Read the model definition and answer for the solid it produces. Units are mm, in the model's axes. Face numbers are marked on the shaded views. A direction names the side the tool comes from. Give positions to 0.01 mm unless a question says otherwise; leave off trailing zeros. Write each loop counter-clockwise with the first axis right and the second up, starting at its lowest first coordinate (ties: lowest second). Pieces come first, ordered by that corner, then holes. Notation, with made-up numbers: (19.5, 74.5) - (29.5, 74.5) arc R20 ccw to (29.5, 83.5) - close; hole circle Ø3 at (23, 16.25). An arc over 180 degrees is marked (long way). Use CSV: the item, a comma, the result in double quotes. Start each with the question number.
from build123d import *

# Parameters (mm, degrees)
RIB1_REACH          = 71.607
SKETCH3_WALL_W      = 156.928914452
SKETCH3_WALL_H      = 8
CHAMFER1_SIZE       = 2
CHAMFER1_SIZE2      = 20
CHAMFER2_SIZE       = 1
CHAMFER2_SIZE2      = 1.144674394
CIRPATTERN23_COUNT  = 4
CUT_EXTRUDE7_REACH  = 71.607
SKETCH5_R           = 1
CIRPATTERN24_COUNT  = 4
SKETCH4_OUTSIDE_W   = 79.882
SKETCH4_OUTSIDE_H   = 79.882
SKETCH4_OUTSIDE_R   = 16.631613782
CUT_EXTRUDE8_DEPTH  = 20
CUT_EXTRUDE8_DRAFT  = -2
SKETCH7_OUTSIDE_W   = 78.484
SKETCH7_OUTSIDE_H   = 78.484
SKETCH7_OUTSIDE_W_2 = 54
SKETCH7_OUTSIDE_H_2 = 56.5
CUT_EXTRUDE9_DEPTH  = 57


with BuildPart() as part:
    # Sketch1 → Revolve1 (revolve)
    with BuildSketch(Plane(origin=(0, 0, 0), x_dir=(0, 0, -1), z_dir=(1, 0, 0))):
        Polygon((10.5, 57), (15.5, 57), (15.921613782, 36.013708049), (16.631613782, 36.013708049), (18.25, 6), (28.25, 6), (28.25, 0), (23.75, 0), (23.75, -3), (19.25, -3), (19.25, 0), (13.75, 0), (13.75, 6.707783598), (12.75, 6.707783598), (12.75, 8.013708049), (11.75, 8.013708049), (11.75, 36.013708049), (10.75, 36.013708049), (10.5, 53), align=None)
    revolve(axis=Axis((0, 0, 0), (0, 1, 0)))

    # Sketch3 wall → Rib1 (add, up to next)
    with BuildSketch(Plane(origin=(22.676470588, 12, 0), x_dir=(0.645690512921, -0.763599215245, 0), z_dir=(0.763599215245, 0.645690512921, 0)), mode=Mode.PRIVATE) as rib1_sk1:
        Rectangle(SKETCH3_WALL_W, SKETCH3_WALL_H)
    rib1_tool1 = extrude(rib1_sk1.sketch, amount=-RIB1_REACH, mode=Mode.PRIVATE) - part.part
    rib1 = rib1_tool1.solids().sort_by_distance((22.676470588, 12, 0))[0]
    add(rib1)

    # Chamfer1
    chamfer1_edges = [part.edges().sort_by_distance(p)[0] for p in [
        (0, 57, 15.5),
    ]]
    chamfer1_side = [part.faces().sort_by_distance(p)[0] for p in [
        (0, 57, 10.938406204),
    ]]
    chamfer(chamfer1_edges, length=CHAMFER1_SIZE, length2=CHAMFER1_SIZE2, reference=chamfer1_side[0])

    # Chamfer2
    chamfer2_edges = [part.edges().sort_by_distance(p)[0] for p in [
        (0, 57, 13.5),
    ]]
    chamfer2_side = [part.faces().sort_by_distance(p)[0] for p in [
        (0, 47.002017422, 14.700859078),
    ]]
    chamfer(chamfer2_edges, length=CHAMFER2_SIZE, length2=CHAMFER2_SIZE2, reference=chamfer2_side[0])

    # CirPattern23: Rib1 ×4 about axis
    cirpattern23_axis = Axis((0, 0, 0), (0, 1, 0))
    for i in range(1, CIRPATTERN23_COUNT):
        add(rib1.rotate(cirpattern23_axis, i * 360 / CIRPATTERN23_COUNT))

    # Sketch5 → Cut-Extrude7 (cut, up to next)
    with BuildSketch(Plane.XZ, mode=Mode.PRIVATE) as cut_extrude7_sk1:
        with Locations(Location((17.67766953, -17.67766953, 0), (0, 0, 270))):
            Circle(SKETCH5_R)
    cut_extrude7_tool1 = extrude(cut_extrude7_sk1.sketch, amount=-CUT_EXTRUDE7_REACH, mode=Mode.PRIVATE) & part.part
    cut_extrude7 = cut_extrude7_tool1.solids().sort_by_distance((17.67767, 0, -17.67767))[0]
    add(cut_extrude7, mode=Mode.SUBTRACT)

    # CirPattern24: Cut-Extrude7 ×4 about axis
    cirpattern24_axis = Axis((0, 0, 0), (0, 1, 0))
    for i in range(1, CIRPATTERN24_COUNT):
        add(cut_extrude7.rotate(cirpattern24_axis, i * 360 / CIRPATTERN24_COUNT), mode=Mode.SUBTRACT)


with BuildPart() as cut_extrude8_tool:
    # Sketch4 outside → Cut-Extrude8 (with draft: the straight prism first)
    with BuildSketch(Plane(origin=(0, 36.013708049, 0), x_dir=(1, 0, 0), z_dir=(0, 1, 0))):
        Rectangle(SKETCH4_OUTSIDE_W, SKETCH4_OUTSIDE_H)
        Circle(SKETCH4_OUTSIDE_R, mode=Mode.SUBTRACT)
    extrude(amount=-CUT_EXTRUDE8_DEPTH)
    # Cut-Extrude8: the draft: its side faces are tilted about the plane it starts from
    cut_extrude8_sides = [cut_extrude8_tool.faces().sort_by_distance(p)[0] for p in [
        (0, 26.013708049, 39.941),
        (39.941, 26.013708049, 0),
        (0, 26.013708049, -39.941),
        (-39.941, 26.013708049, 0),
        (-16.631613782, 26.013708049, 0),
    ]]
    draft(cut_extrude8_sides, Plane(origin=(0, 36.013708049, 0), x_dir=(1, 0, 0), z_dir=(0, 1, 0)), CUT_EXTRUDE8_DRAFT)


with BuildPart() as part_1:
    add(part.part)

    # Cut-Extrude8: cut by cut_extrude8_tool
    add(cut_extrude8_tool.part, mode=Mode.SUBTRACT)

    # Sketch7 outside → Cut-Extrude9 (cut)
    with BuildSketch(Plane(origin=(0, 0, 0), x_dir=(1, 0, 0), z_dir=(0, 1, 0))):
        Rectangle(SKETCH7_OUTSIDE_W, SKETCH7_OUTSIDE_H)
        Rectangle(SKETCH7_OUTSIDE_W_2, SKETCH7_OUTSIDE_H_2, mode=Mode.SUBTRACT)
    extrude(amount=CUT_EXTRUDE9_DEPTH, mode=Mode.SUBTRACT)


solid = part_1.part
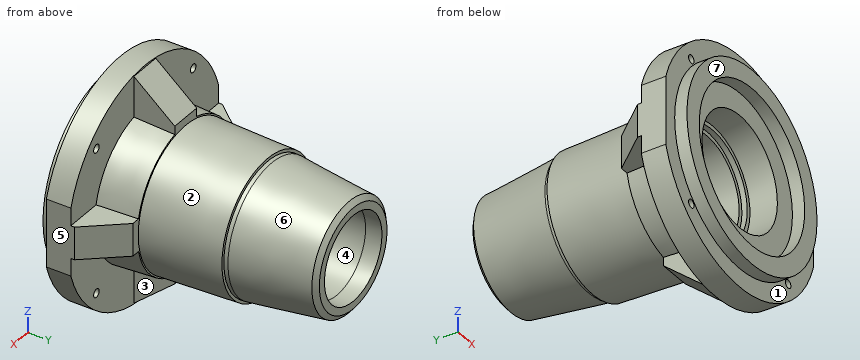
(1) Which of the six approach directions +Z, -Z, +X, -X, +Y, -Y give full straight-line access (tool end or side, diameter ignored) to the marked faces 1, 2 and 3?
(2) The part is cut by section B-B on y = 17. Write down the section's boundary in (x, z).
(3) Given P1, Ø1.8, axis at x = -17.68, z = 17.68, coming from the +Y side; P2, Ø2, axis at y = 27.5, z = -16, coming from the +X side; P3, Ø8, axis at y = 20.5, z = -8.5, coming from the +X side; P4, Ø8, axis at x = -14.5, z = 9, coming from the +Y side, each flat-ended and moving along its own axis, determine where each tip first touches the part or whether it passes through.
(4) Consider probe 1 along Z at (x, y) = (0, 3.25); probe 2 along Y at (x, z) = (9, -15); probe 3 along Z at (x, y) = (0, 7.05). Determine where each line is inside the solid, lowest interval first.
(5) For a pull along X with two mould halves and no side action, classify the marked faces 4, 5, 6 and 7 as pulls with the +X half, pulls with the -X half, needs draft (parallel to the pull), parting line crosses it, or undercut.
(6) The part is cut by section C-C on y = 40. Write down the section's boundary in (x, z), plus the area to 3 significant figures.
(7) The part is cut by section A-A on y = 10.5. Write down the section's boundary in (x, z).
Reported:
1,face 1,"-Y"
1,face 2,"+Y"
1,face 3,"-Z, +X, +Y"
2,outline,"circle Ø34.59 at (0, 0); hole circle Ø23.5 at (0, 0)"
3,P1,"through"
3,P2,"x = 7.85"
3,P3,"x = 16.58"
3,P4,"y = 56.44"
4,probe 1,"-28.25 to -13.75, 13.75 to 28.25"
4,probe 2,"0 to 16.01"
4,probe 3,"-26.86 to -12.75, 12.75 to 26.86"
5,face 4,"undercut"
5,face 5,"pulls with the +X half"
5,face 6,"parting line crosses it"
5,face 7,"needs draft"
6,outline,"circle Ø31.08 at (0, 0); hole circle Ø21.38 at (0, 0)"
6,area,"400 mm²"
7,outline,"(-23.94, -4) - (-17.56, -4) arc R18.01 ccw to (-4, -17.56) - (-4, -23.94) - (4, -23.94) - (4, -17.56) arc R18.01 ccw to (17.56, -4) - (23.94, -4) - (23.94, 4) - (17.56, 4) arc R18.01 ccw to (4, 17.56) - (4, 23.94) - (-4, 23.94) - (-4, 17.56) arc R18.01 ccw to (-17.56, 4) - (-23.94, 4) - close; hole circle Ø23.5 at (0, 0)"
